Verification items for the finished model (mm, model axes). A direction names the side the tool comes from. Coordinates: 2 decimals unless noted, no trailing zeros. Order: outer loops, then holes, each group sorted by start corner. A loop starts at its lowest first (then second) coordinate and runs counter-clockwise, first axis right, second up.
Q1. Cross-section at B-B, the plane z = -24. Record the boundary of the cut face in (x, y).
Q2. Set-up check for faces 1 (the flat face through (115.1, 62, -37)), 2 (the cylindrical face through (81.831, 28.418, -25.417)), 3 (the flat face through (101, 50, -29)), 4 (the flat face through (80, 50, -38)), 5 (the flat face through (99, 50, -39)): record each of +Z, -Z, +X, -X, +Y, -Y from which the full face is reachable in a straight line by a thin tool's end or side.
Q3. Cross-section at D-D, the plane y = 24.5. Record the boundary of the cut face in (x, z).
Q4. Cross-section at A-A, the plane x = 82. Record the boundary of the cut face in (y, z).
Q5. Depth check by flat-ended pin: P1, Ø4, axis at x = 104.5, y = 61.5, coming from the +Z side; P2, Ø1.6, axis at x = 79, y = 63.5, coming from the -Z side; P3, Ø6, axis at y = 24.5, z = -24, coming from the +X side. Enter the tip coordinate at first touch or a pass-through.
Q6. Cross-section at C-C, the plane z = -12. Record the boundary of the cut face in (x, y).
Q7. Draft check along Z on faces 6 (the flat face through (81, 50, 15)), 7 (the flat face through (79.6, 77, 4)), 8 (the flat face through (92.33, 40.6, -36.78)). Enter one of: pulls with the +Z half, pulls with the -Z half, needs draft (parallel to the pull), parting line crosses it, or undercut.
Q8. Thickness scan on line 1 (Z direction, x = 83.1, y = 25); line 2 (X direction, y = 62.5, z = -32.4); line 3 (Y direction, x = 102, z = -39.5). Record the ranges inside material, lowest first.
from build123d import *

# Parameters (mm, degrees)
PAD_DEPTH        = 62
HOLE_D           = 4.5
HOLE_DEPTH       = 25
HOLE_CBORE_D     = 7.4
HOLE_CBORE_DEPTH = 4.4
SKETCH069_R      = 2.25
HOLE006_DEPTH    = 60.001
POCKET022_DEPTH  = 4.5
SKETCH071_W      = 40
SKETCH071_H      = 40
POCKET023_DEPTH  = 8
CHAMFER_SIZE     = 3
CHAMFER018_SIZE  = 3


with BuildPart() as part:
    # Sketch → Pad (new body)
    with BuildSketch(Plane.XZ.offset(-19)):
        Polygon((76, 15), (76, -35), (78, -35), (78, -47), (116, -47), (116, -29), (82, -29), (82, 15), align=None)
    extrude(amount=-PAD_DEPTH)

    # Hole
    with Locations(Plane.YZ.offset(82)):
        with Locations((25, -24), (25, 6), (41, 8), (41, -12), (75, 6), (75, -24)):
            CounterBoreHole(HOLE_D / 2, HOLE_CBORE_D / 2, HOLE_CBORE_DEPTH, depth=HOLE_DEPTH)

    # Sketch069 → Hole006 (cut, through all)
    with BuildSketch(Plane.XY.offset(-45)):
        with Locations((88.5, 62.5)):
            Circle(SKETCH069_R)
        with Locations((109.5, 37.5)):
            Circle(SKETCH069_R)
        with Locations((109.5, 62.5)):
            Circle(SKETCH069_R)
        with Locations((88.5, 37.5)):
            Circle(SKETCH069_R)
    extrude(amount=HOLE006_DEPTH, mode=Mode.SUBTRACT)

    # Sketch070 → Pocket022 (cut)
    with BuildSketch(Plane.XY.offset(-39)):
        Polygon((92.1, 64.578461), (88.5, 66.656922), (84.9, 64.578461), (84.9, 60.421539), (88.5, 58.343078), (92.1, 60.421539), align=None)
        Polygon((113.1, 64.578461), (109.5, 66.656922), (105.9, 64.578461), (105.9, 60.421539), (109.5, 58.343078), (113.1, 60.421539), align=None)
        Polygon((113.1, 39.578461), (109.5, 41.656922), (105.9, 39.578461), (105.9, 35.421539), (109.5, 33.343078), (113.1, 35.421539), align=None)
        Polygon((92.1, 39.578461), (88.5, 41.656922), (84.9, 39.578461), (84.9, 35.421539), (88.5, 33.343078), (92.1, 35.421539), align=None)
    extrude(amount=POCKET022_DEPTH, mode=Mode.SUBTRACT)

    # Sketch071 → Pocket023 (cut)
    with BuildSketch(Plane.XY.offset(-47)):
        with Locations((96, 50)):
            Rectangle(SKETCH071_W, SKETCH071_H)
    extrude(amount=POCKET023_DEPTH, mode=Mode.SUBTRACT)

    # Chamfer
    chamfer_edges = [part.edges().sort_by_distance(p)[0] for p in [
        (116, 81, -38),
    ]]
    chamfer(chamfer_edges, length=CHAMFER_SIZE)

    # Chamfer018
    chamfer018_edges = [part.edges().sort_by_distance(p)[0] for p in [
        (116, 19, -38),
    ]]
    chamfer(chamfer018_edges, length=CHAMFER018_SIZE)


with BuildPart() as part_1:
    # Body placement: moved
    add(part.part.moved(Location((2, 0, 0))))


solid = part_1.part
Check values:
1. outline: (78, 19) - (84, 19) - (84, 21.3) - (79.6, 21.3) - (79.6, 22.75) - (78, 22.75) - close; (78, 27.25) - (79.6, 27.25) - (79.6, 28.7) - (84, 28.7) - (84, 71.3) - (79.6, 71.3) - (79.6, 72.75) - (78, 72.75) - close; (78, 77.25) - (79.6, 77.25) - (79.6, 78.7) - (84, 78.7) - (84, 81) - (78, 81) - close
2. face 1: -Z
2. face 2: +X
2. face 3: +Z, +X, +Y, -Y
2. face 4: -Z, -X, +Y, -Y
2. face 5: -Z, +X, -X
3. outline: (78, -35) - (80, -35) - (80, -47) - (118, -47) - (118, -29) - (84, -29) - (84, -27.67) - (79.6, -27.67) - (79.6, -26.19) - (78, -26.19) - close; (78, -21.81) - (79.6, -21.81) - (79.6, -20.33) - (84, -20.33) - (84, 2.33) - (79.6, 2.33) - (79.6, 3.81) - (78, 3.81) - close; (78, 8.19) - (79.6, 8.19) - (79.6, 9.67) - (84, 9.67) - (84, 15) - (78, 15) - close
4. outline: (19, -47) - (30, -47) - (30, -39) - (70, -39) - (70, -47) - (81, -47) - (81, 15) - (19, 15) - close; hole circle Ø7.4 at (25, -24); hole circle Ø7.4 at (25, 6); hole circle Ø7.4 at (41, -12); hole circle Ø7.4 at (41, 8); hole circle Ø7.4 at (75, -24); hole circle Ø7.4 at (75, 6)
5. P1: stops at z = -29
5. P2: stops at z = -35
5. P3: stops at x = 79.6
6. outline: (78, 19) - (84, 19) - (84, 37.3) - (79.6, 37.3) - (79.6, 38.75) - (78, 38.75) - close; (78, 43.25) - (79.6, 43.25) - (79.6, 44.7) - (84, 44.7) - (84, 81) - (78, 81) - close
7. face 6: pulls with the +Z half
7. face 7: undercut
7. face 8: needs draft
8. line 1: z = -47 to -27.7, -20.3 to 2.3, 9.7 to 15
8. line 2: x = 78 to 88.25, 92.75 to 109.25, 113.75 to 118
8. line 3: y = 19 to 30, 70 to 81
